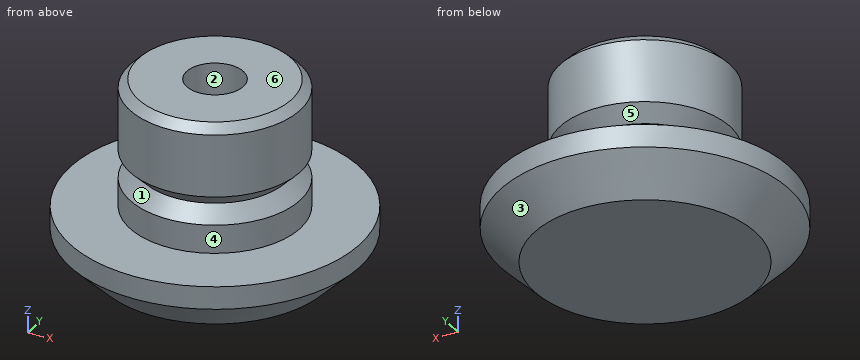
from build123d import *

# Parameters (mm, degrees)
F2_SIZE = 0.3
F3_SIZE = 0.49999
F4_SIZE = 1.2


# Not quite as in the source:
# - a fillet or chamfer is up to 0.001 mm smaller than in the source, because OpenCascade refuses the exact size


with BuildPart() as f1:
    # F0 (on Front) → F1 (revolve)
    with BuildSketch(Plane.XZ):
        Polygon((5.1, -2), (5.1, 0), (3, 0), (3, 1), (2.5, 1), (2.5, 2), (3, 2), (3, 4.5), (1, 4.5), (1, 2), (0, 2), (0, 0), (0, -2), align=None)
    revolve(axis=Axis((0, 0, -1), (0, 0, -1)))

    # F2
    f2_edges = [f1.edges().sort_by_distance(p)[0] for p in [
        (-3, 0, 4.5),
    ]]
    chamfer(f2_edges, length=F2_SIZE)

    # F3 (size 0.5 in the source; OpenCascade refuses exactly that, so slightly less here)
    f3_edges = [f1.edges().sort_by_distance(p)[0] for p in [
        (-2.5, 0, 2),
        (-2.5, 0, 1),
    ]]
    chamfer(f3_edges, length=F3_SIZE)

    # F4
    f4_edges = [f1.edges().sort_by_distance(p)[0] for p in [
        (-5.1, 0, -2),
    ]]
    chamfer(f4_edges, length=F4_SIZE)


solid = f1.part
Input: part model. Units: mm. Frame: model coordinates. Face numbers are marked on the shaded views. A direction names the side the tool comes from. Round coordinates to 2 decimals unless told otherwise and drop trailing zeros. Order: outer loops, then holes, each group sorted by start corner. A loop starts at its lowest first (then second) coordinate and runs counter-clockwise, first axis right, second up. Notation, with made-up numbers: (-16, -19) - (5, -19) arc R29 cw to (5, 19) - close; hole circle Ø2 at (13.25, 39). An arc over 180 degrees is marked (long way). Use a Markdown table: item, result.
1. Access query for the marked faces 4, 5 and 6. Directions: +Z, -Z, +X, -X, +Y, -Y. A direction counts if a zero-diameter tool reaches every point of the face in a straight line with its end or side. Return the directions, or none.
Evaluation:
| item | result |
|---|---|
| face 4 | +Z |
| face 5 | none |
| face 6 | +Z, +X, -X, +Y, -Y |
2. Mould query, pull axis Z, two halves, no side actions, for the marked faces 1, 2 and 3. Classes: +Z half, -Z half, draft (parallel to the pull), parting line (faces both ways), or undercut.
Evaluation:
| item | result |
|---|---|
| face 1 | undercut |
| face 2 | draft |
| face 3 | -Z half |
3. Material intervals for probe 1 along Y at (x, z) = (0, 3.15); probe 2 along Z at (x, y) = (1.5, -3), sorted ascending.
Evaluation:
| item | result |
|---|---|
| probe 1 | -3 to -1, 1 to 3 |
| probe 2 | -2 to 0 |
4. Section C-C on z = -0.5. Return the cut outline in (x, y), then the cut area to 3 significant figures.
Evaluation:
| item | result |
|---|---|
| outline | circle Ø10.2 at (0, 0) |
| area | 81.7 mm^2 |
5. Section D-D on z = 1.25. Return the cut outline in (x, y), then the cut area to 3 significant figures.
Evaluation:
| item | result |
|---|---|
| outline | circle Ø5.5 at (0, 0) |
| area | 23.8 mm^2 |
